from build123d import *

# Parameters (mm, degrees)
SKETCH1_R           = 31.75
BOSS_EXTRUDE1_DEPTH = 6.35
SKETCH2_R           = 12.7
SKETCH2_R_2         = 2.5527
CUT_EXTRUDE1_DEPTH  = 7.35
SKETCH3_R           = 15.875
SKETCH3_R_2         = 12.7
BOSS_EXTRUDE2_DEPTH = 2.54


with BuildPart() as part:
    # Sketch1 → Boss-Extrude1 (new body)
    with BuildSketch(Plane.XY):
        Circle(SKETCH1_R)
    extrude(amount=BOSS_EXTRUDE1_DEPTH)

    # Sketch2 → Cut-Extrude1 (cut, through all)
    with BuildSketch(Plane.XY.offset(6.35)):
        Circle(SKETCH2_R)
        with Locations((0, 23.8125)):
            Circle(SKETCH2_R_2)
        with Locations((20.622229928, 11.90625)):
            Circle(SKETCH2_R_2)
        with Locations((20.622229928, -11.90625)):
            Circle(SKETCH2_R_2)
        with Locations((0, -23.8125)):
            Circle(SKETCH2_R_2)
        with Locations((-20.622229928, -11.90625)):
            Circle(SKETCH2_R_2)
        with Locations((-20.622229928, 11.90625)):
            Circle(SKETCH2_R_2)
    extrude(amount=-CUT_EXTRUDE1_DEPTH, mode=Mode.SUBTRACT)

    # Sketch3 → Boss-Extrude2 (add)
    with BuildSketch(Plane.XY.offset(6.35)):
        Circle(SKETCH3_R)
        Circle(SKETCH3_R_2, mode=Mode.SUBTRACT)
    extrude(amount=BOSS_EXTRUDE2_DEPTH)


solid = part.part
Can you work these out from the model? Positions are in its coordinate system, mm. A direction names the side the tool comes from. Coordinates: 2 decimals unless noted, no trailing zeros. Write each loop counter-clockwise with the first axis right and the second up, starting at its lowest first coordinate (ties: lowest second). Pieces come first, ordered by that corner, then holes. Notation, with made-up numbers: (43, 37) -> (50, 37) arc R30 cw to (50, 66) -> close; hole circle Ø9 at (35.25, 61.25). An arc over 180 degrees is marked (long way). Write item = value, one per line.
(1) If I drill on probe 1 along Y at (x, z) = (0, 4.75); probe 2 along X at (y, z) = (-13.5, 3.5); probe 3 along Y at (x, z) = (-2, 6), over which ranges is the centre line in solid material (lowest first)?
Verdict:
probe_1 = -31.75 to -26.37, -21.26 to -12.7, 12.7 to 21.26, 26.37 to 31.75
probe_2 = -28.74 to -22.62, -18.63 to 18.63, 22.62 to 28.74
probe_3 = -31.69 to -25.4, -22.23 to -12.54, 12.54 to 22.23, 25.4 to 31.69
(2) Imagine slicing it at B-B (x = 0). Please give me the cut outline in (y, z) (3 decimals).
Verdict:
outline = (-31.75, 0) -> (-26.365, 0) -> (-26.365, 6.35) -> (-31.75, 6.35) -> close; (-21.26, 0) -> (-12.7, 0) -> (-12.7, 8.89) -> (-15.875, 8.89) -> (-15.875, 6.35) -> (-21.26, 6.35) -> close; (12.7, 0) -> (21.26, 0) -> (21.26, 6.35) -> (15.875, 6.35) -> (15.875, 8.89) -> (12.7, 8.89) -> close; (26.365, 0) -> (31.75, 0) -> (31.75, 6.35) -> (26.365, 6.35) -> close
(3) Imagine slicing it at A-A (y = 0). Please give me the cut outline in (x, z) (3 decimals).
Verdict:
outline = (-31.75, 0) -> (-12.7, 0) -> (-12.7, 8.89) -> (-15.875, 8.89) -> (-15.875, 6.35) -> (-31.75, 6.35) -> close; (12.7, 0) -> (31.75, 0) -> (31.75, 6.35) -> (15.875, 6.35) -> (15.875, 8.89) -> (12.7, 8.89) -> close
(4) For pin 1 (6.5 mm diameter, centred on x = -20.62, y = 11.91, fed in from +Z); pin 2 (1.5 mm diameter, centred on y = 10, z = 2.5, fed in from +X); pin 3 (4 mm diameter, centred on x = 20.62, y = -11.91, fed in from -Z); pin 4 (4 mm diameter, centred on y = -18, z = 1, fed in from +X), each with a flat end and sliding along its axis, tell me the tip position at first contact or that it passes through.
Verdict:
pin_1 = 6.35
pin_2 = 30.37
pin_3 = through
pin_4 = 27.42
(5) Imagine slicing it at D-D (z = 7.5). Please give me the cut outline in (x, y) (3 decimals), and give its area (3 significant figures).
Verdict:
outline = circle Ø31.75 at (0, 0); hole circle Ø25.4 at (0, 0)
area = 285 mm^2
(6) Imagine slicing it at C-C (x = -10.5). Please give me the cut outline in (y, z).
Verdict:
outline = (-29.96, 0) -> (-7.14, 0) -> (-7.14, 8.89) -> (-11.91, 8.89) -> (-11.91, 6.35) -> (-29.96, 6.35) -> close; (7.14, 0) -> (29.96, 0) -> (29.96, 6.35) -> (11.91, 6.35) -> (11.91, 8.89) -> (7.14, 8.89) -> close
(7) On a 3-axis mill with a long thin cutter (end or side, diameter ignored), from which of +Z, -Z, +X, -X, +Y, -Y can I reach the whole of each face in a straight line? I mean faces 1 (the face through (-3.441, -15.497, 7.602)), 2 (the face through (1.372, 25.965, 3.219)). Say none if no direction works.
Verdict:
face_1 = +Z
face_2 = +Z, -Z
(8) Thinking about a two-plate mould opening in Y: for faces 3 (the face through (14, 0, 0)), 4 (the face through (-6.883, -30.995, 3.131)), 5 (the face through (1.37, -21.66, 3.22)), which applies, +Y half, -Y half, draft (parallel to the pull), parting line (faces both ways), or undercut?
Verdict:
face_3 = draft
face_4 = parting line
face_5 = undercut
